Read the model definition and answer for the solid it produces. Units are mm, in the model's axes. Coordinates: 2 decimals unless noted, no trailing zeros. Write each loop counter-clockwise with the first axis right and the second up, starting at its lowest first coordinate (ties: lowest second). Pieces come first, ordered by that corner, then holes. Notation, with made-up numbers: (72.25, 56) -> (104.25, 56) arc R10 ccw to (104.25, 66) -> close; hole circle Ø8 at (-1, 49.5). An arc over 180 degrees is marked (long way). Return JSON: item names as keys, results as strings.
from build123d import *

# Parameters (mm, degrees)
SKETCH_1_W             = 1.5
SKETCH_1_H             = 186
SM_BASE_FLANGE_1_DEPTH = 130
SKETCH_6_R             = 2.75
CUT_EXTRUDE_1_DEPTH    = 227.932258615
CUT_EXTRUDE_2_DEPTH    = 10
CUT_EXTRUDE_4_DEPTH    = 10
EXTRUDE_1_DEPTH        = 1.5


# Sheet-metal steps are written as plain solids
with BuildPart() as part:
    # Sketch 1 → 基体-法兰1 (new body)
    with BuildSketch(Plane.XY):
        with Locations((0.75, 93)):
            Rectangle(SKETCH_1_W, SKETCH_1_H)
    extrude(amount=SM_BASE_FLANGE_1_DEPTH)

    # 草图6 → 切除-拉伸1 (cut, through all)
    with BuildSketch(Plane.ZY):
        with Locations((5, 153)):
            Circle(SKETCH_6_R)
        with Locations((5, 93)):
            Circle(SKETCH_6_R)
        with Locations(Location((5, 33, 0), (0, 0, 180))):
            Circle(SKETCH_6_R)
    extrude(amount=-CUT_EXTRUDE_1_DEPTH, mode=Mode.SUBTRACT)

    # 草图7 → 切除-拉伸2 (cut)
    with BuildSketch(Plane(origin=(1.5, 0, 0), x_dir=(0, 0, -1), z_dir=(1, 0, 0))):
        Polygon((-14.94, 186), (-130, 186), (-130, -13.441807708), align=None)
    extrude(amount=-CUT_EXTRUDE_2_DEPTH, mode=Mode.SUBTRACT)

    # 草图8 → 切除-拉伸4 (cut)
    with BuildSketch(Plane.ZY):
        Polygon((122.245284915, 0), (110.646921999, 20.104280083), (75.798721386, 0), align=None)
    extrude(amount=-CUT_EXTRUDE_4_DEPTH, mode=Mode.SUBTRACT)

    # 草图10 → 凸台-拉伸1 (add)
    with BuildSketch(Plane(origin=(1.5, 0, 0), x_dir=(0, 0, -1), z_dir=(1, 0, 0))):
        Polygon((-75.798721386, 0), (0, 0), (0, -43.729050508), align=None)
    extrude(amount=-EXTRUDE_1_DEPTH)


solid = part.part
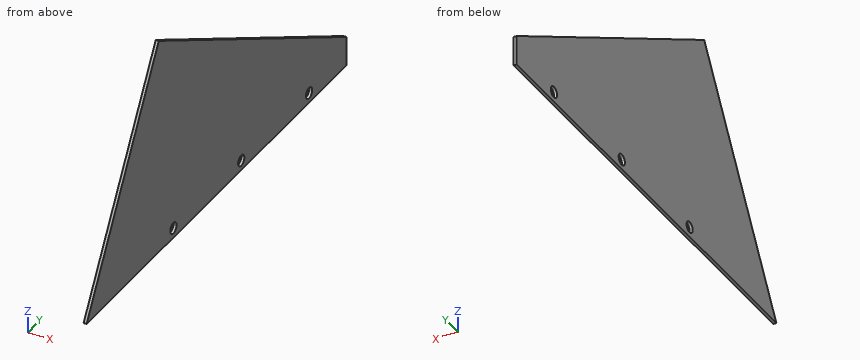
1. The part is cut by section B-B (y = 33). Determine the outline of the cut face in (x, z).
Taken from the geometry:
{"outline": "(0, 0) -> (1.5, 0) -> (1.5, 2.25) -> (0, 2.25) -> close; (0, 7.75) -> (1.5, 7.75) -> (1.5, 103.21) -> (0, 103.21) -> close"}
2. Consider L1, parallel to Y at x = 0.95, z = 5; L2, parallel to Z at x = 0.6, y = 153; L3, parallel to Z at x = 1.1, y = 33. Determine where each line is inside the solid, lowest interval first.
Taken from the geometry:
{"L1": "y = -40.84 to 30.25, 35.75 to 90.25, 95.75 to 150.25, 155.75 to 186", "L2": "z = 0 to 2.25, 7.75 to 33.98", "L3": "z = 0 to 2.25, 7.75 to 103.21"}
3. The part is cut by section D-D (y = 153). Determine the outline of the cut face in (x, z), then the cut area to 3 significant figures.
Taken from the geometry:
{"outline": "(0, 0) -> (1.5, 0) -> (1.5, 2.25) -> (0, 2.25) -> close; (0, 7.75) -> (1.5, 7.75) -> (1.5, 33.98) -> (0, 33.98) -> close", "area": "42.7 mm2"}
4. The part is cut by section A-A (z = 5). Determine the outline of the cut face in (x, y), then the cut area to 3 significant figures.
Taken from the geometry:
{"outline": "(0, -40.84) -> (1.5, -40.84) -> (1.5, 30.25) -> (0, 30.25) -> close; (0, 35.75) -> (1.5, 35.75) -> (1.5, 90.25) -> (0, 90.25) -> close; (0, 95.75) -> (1.5, 95.75) -> (1.5, 150.25) -> (0, 150.25) -> close; (0, 155.75) -> (1.5, 155.75) -> (1.5, 186) -> (0, 186) -> close", "area": "316 mm2"}
5. The part is cut by section C-C (x = 1). Determine the outline of the cut face in (y, z).
Taken from the geometry:
{"outline": "(-43.73, 0) -> (186, 0) -> (186, 14.94) -> (20.1, 110.65) -> close; hole circle Ø5.5 at (33, 5); hole circle Ø5.5 at (93, 5); hole circle Ø5.5 at (153, 5)"}
